from build123d import *

# Parameters (mm, degrees)
SKETCH_1_R          = 65
EXTRUDE_1_DEPTH     = 5
SKETCH_2_R          = 59.85
EXTRUDE_2_DEPTH     = 3
SKETCH_3_W          = 35
SKETCH_3_H          = 30
EXTRUDE_3_DEPTH     = 25
SKETCH_5_R          = 4.1
CUT_EXTRUDE_2_DEPTH = 96.262794416
SKETCH_6_R          = 2.75
CUT_EXTRUDE_3_DEPTH = 98.667804316
SKETCH2_W           = 20.25
SKETCH2_H           = 10.35
CUT_EXTRUDE1_DEPTH  = 108.964114408
CHAMFER1_SIZE       = 2
CHAMFER1_SIZE2      = 0.535898385
SKETCH4_W           = 35
SKETCH4_H           = 30
CUT_EXTRUDE3_DEPTH  = 12.5
BOSS_EXTRUDE2_START = -2
SKETCH5_W           = 20
SKETCH5_H           = 70
BOSS_EXTRUDE2_DEPTH = 5.325
SKETCH6_R           = 4.15
CUT_EXTRUDE4_DEPTH  = 93.884636108
CUT_EXTRUDE5_DEPTH  = 6.5
CHAMFER2_SIZE       = 1
CHAMFER2_SIZE2      = 2.747477419
SKETCH8_W           = 17.5
SKETCH8_H           = 27.9
CUT_EXTRUDE6_DEPTH  = 5


with BuildPart() as part:
    # Эскиз1 → Бобышка-Вытянуть1 (new body)
    with BuildSketch(Plane(origin=(0, 0, 0), x_dir=(1, 0, 0), z_dir=(0, 1, 0))):
        with Locations(Location((0, 0, 0), (0, 0, 270))):
            Circle(SKETCH_1_R)
    extrude(amount=EXTRUDE_1_DEPTH)

    # Эскиз2 → Бобышка-Вытянуть2 (add)
    with BuildSketch(Plane(origin=(0, 5, 0), x_dir=(1, 0, 0), z_dir=(0, 1, 0))):
        with Locations(Location((0, 0, 0), (0, 0, 270))):
            Circle(SKETCH_2_R)
    extrude(amount=EXTRUDE_2_DEPTH)

    # Эскиз3 → Бобышка-Вытянуть3 (add)
    with BuildSketch(Plane.XZ):
        Rectangle(SKETCH_3_W, SKETCH_3_H)
    extrude(amount=EXTRUDE_3_DEPTH)

    # Эскиз5 → Вырез-Вытянуть2 (cut, through all)
    with BuildSketch(Plane.XZ):
        with Locations(Location((33.234018716, -33.234018716, 0), (0, 0, 270))):
            Circle(SKETCH_5_R)
        with Locations(Location((-33.234018716, -33.234018716, 0), (0, 0, 270))):
            Circle(SKETCH_5_R)
        with Locations(Location((-33.234018716, 33.234018716, 0), (0, 0, 270))):
            Circle(SKETCH_5_R)
        with Locations(Location((33.234018716, 33.234018716, 0), (0, 0, 270))):
            Circle(SKETCH_5_R)
    extrude(amount=-CUT_EXTRUDE_2_DEPTH, mode=Mode.SUBTRACT)

    # Эскиз6 → Вырез-Вытянуть3 (cut, through all)
    with BuildSketch(Plane(origin=(0, 8, 0), x_dir=(1, 0, 0), z_dir=(0, 1, 0))):
        with Locations(Location((-18, 20, 0), (0, 0, 270))):
            Circle(SKETCH_6_R)
    extrude(amount=-CUT_EXTRUDE_3_DEPTH, mode=Mode.SUBTRACT)

    # Sketch2 → Cut-Extrude1 (cut, through all)
    with BuildSketch(Plane.ZY.offset(17.5)):
        with Locations((0, -12.5)):
            Rectangle(SKETCH2_W, SKETCH2_H)
    extrude(amount=-CUT_EXTRUDE1_DEPTH, mode=Mode.SUBTRACT)

    # Chamfer1
    chamfer1_edges = [part.edges().sort_by_distance(p)[0] for p in [
        (0, 8, -59.85),
    ]]
    chamfer1_side = [part.faces().sort_by_distance(p)[0] for p in [
        (0, 6.5, -59.85),
    ]]
    chamfer(chamfer1_edges, length=CHAMFER1_SIZE, length2=CHAMFER1_SIZE2, reference=chamfer1_side[0])

    # Sketch4 → Cut-Extrude3 (cut)
    with BuildSketch(Plane.XZ.offset(25)):
        Rectangle(SKETCH4_W, SKETCH4_H)
    extrude(amount=-CUT_EXTRUDE3_DEPTH, mode=Mode.SUBTRACT)

    # Sketch5 → Boss-Extrude2 (add)
    with BuildSketch(Plane.XZ.offset(7.325).offset(BOSS_EXTRUDE2_START)):
        Rectangle(SKETCH5_W, SKETCH5_H)
    extrude(amount=-BOSS_EXTRUDE2_DEPTH)

    # Sketch6 → Cut-Extrude4 (cut, through all)
    with BuildSketch(Plane.XZ.offset(5.325)):
        with Locations(Location((0, 25, 0), (0, 0, 270))):
            Circle(SKETCH6_R)
        with Locations(Location((0, -25, 0), (0, 0, 270))):
            Circle(SKETCH6_R)
    extrude(amount=-CUT_EXTRUDE4_DEPTH, mode=Mode.SUBTRACT)

    # Sketch7 → Cut-Extrude5 (cut)
    with BuildSketch(Plane(origin=(0, 8, 0), x_dir=(1, 0, 0), z_dir=(0, 1, 0))):
        Polygon((0, -32.5), (6.495190528, -28.75), (6.495190528, -21.25), (0, -17.5), (-6.495190528, -21.25), (-6.495190528, -28.75), align=None)
        Polygon((0, 17.5), (6.495190528, 21.25), (6.495190528, 28.75), (0, 32.5), (-6.495190528, 28.75), (-6.495190528, 21.25), align=None)
    extrude(amount=-CUT_EXTRUDE5_DEPTH, mode=Mode.SUBTRACT)

    # Chamfer2
    chamfer2_edges = [part.edges().sort_by_distance(p)[0] for p in [
        (-3.247595264, 8, 30.625),
        (3.247595264, 8, 30.625),
        (6.495190528, 8, 25),
        (3.247595264, 8, 19.375),
        (-3.247595264, 8, 19.375),
        (-6.495190528, 8, 25),
        (-3.247595264, 8, -19.375),
        (3.247595264, 8, -19.375),
        (6.495190528, 8, -25),
        (3.247595264, 8, -30.625),
        (-3.247595264, 8, -30.625),
        (-6.495190528, 8, -25),
    ]]
    chamfer2_side = [part.faces().sort_by_distance(p)[0] for p in [
        (0.040630406, 8, 0.045144896),
    ]]
    chamfer(chamfer2_edges, length=CHAMFER2_SIZE, length2=CHAMFER2_SIZE2, reference=chamfer2_side[0])

    # Sketch8 → Cut-Extrude6 (cut)
    with BuildSketch(Plane(origin=(0, 8, 0), x_dir=(1, 0, 0), z_dir=(0, 1, 0))):
        with Locations((-35, -2)):
            Rectangle(SKETCH8_W, SKETCH8_H)
    extrude(amount=-CUT_EXTRUDE6_DEPTH, mode=Mode.SUBTRACT)


solid = part.part
Read the model definition and answer for the solid it produces. Units are mm, in the model's axes. A direction names the side the tool comes from. Give positions to 0.01 mm unless a question says otherwise; leave off trailing zeros. Loops run counter-clockwise (first coordinate to the right, second up) from the corner with the lowest first, then second, coordinate; pieces in that order, holes last. Notation, with made-up numbers: M -35,11 L -3,11 A11 cw -3,30 Z; hole C -37,25.5 d8. An arc over 180 degrees is marked long. Write each question's results on one line, items separated by ' | '.
1. Section A-A on y = -9.5 is taken. Give the vertices of the cut face in (x, z) (3 decimals).
Values:
outline: M -17.5,-15 L 17.5,-15 L 17.5,-10.125 L -17.5,-10.125 Z; M -17.5,10.125 L 17.5,10.125 L 17.5,15 L -17.5,15 Z
2. Given pin 1 (5.5 mm diameter, centred on x = -38, y = 5.5, fed in from -Z); pin 2 (10 mm diameter, centred on x = 3, z = 24, fed in from -Y) (3 decimals); pin 3 (8 mm diameter, centred on y = 3.5, z = -25, fed in from -X), each flat-ended and moving along its own axis, determine where each tip first touches the part or whether it passes through.
Values:
pin 1: stops at z = -54.58 | pin 2: stops at y = -5.325 | pin 3: stops at x = -61.51
3. Section B-B on y = -1.75 is taken. Give the vertices of the cut face in (x, z), plus the area to 3 significant figures.
Values:
outline: M -17.5,-15 L -10,-15 L -10,-35 L 10,-35 L 10,-15 L 17.5,-15 L 17.5,15 L 10,15 L 10,35 L -10,35 L -10,15 L -17.5,15 Z; hole C 0,-25 d8.3; hole C 0,25 d8.3 | area: 1,740 mm^2
4. The mould has two halves that part along Z. Classify faces 4 (the face through (3.442, 6.607, 31.082)), 5 (the face through (-13.5, 0, -15.4)): pulls with the +Z half, pulls with the -Z half, needs draft (parallel to the pull), parting line crosses it, or undercut.
Values:
face 4: undercut | face 5: needs draft
5. A tool of negligible diameter and unlimited length cuts with its end or side. For faces 1 (the face through (-32.002, 3.944, -37.145)), 2 (the face through (3.55, 6.61, 18.98)), 3 (the face through (0, -10, 10.125)), from which of +Z, -Z, +X, -X, +Y, -Y can it reach the whole face along a straight path? Write none if from no direction.
Values:
face 1: +Y, -Y | face 2: +Y | face 3: +X, -X, -Y
6. Straight lines are drawn through the part: line 1 (X direction, y = -1.5, z = 25); line 2 (Y direction, x = 1, z = 3.5) (3 decimals); line 3 (Z direction, x = 34, y = 0.5). For each, find the intervals that lie inside material, in ascending order. Write a range as [from, to].
Values:
line 1: x = [-10, -4.15], [4.15, 10] | line 2: y = [-7.325, 8] | line 3: z = [-55.4, -37.26], [-29.21, 29.21], [37.26, 55.4]
